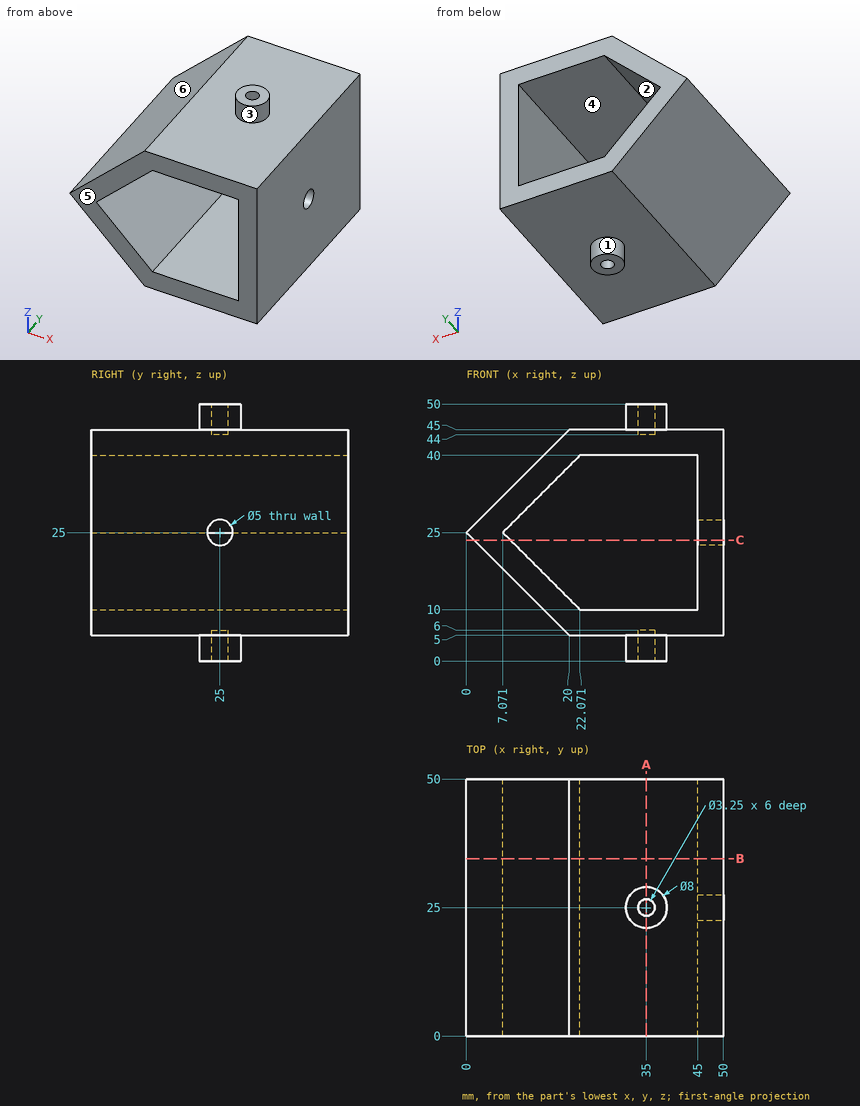
Verification items for this drawing (mm, ordinates from the low corner). A direction names the side the tool comes from. Give positions to 0.01 mm unless a question says otherwise; leave off trailing zeros. Loops run counter-clockwise (first coordinate to the right, second up) from the corner with the lowest first, then second, coordinate; pieces in that order, holes last.
1. Cross-section at A-A on x = 35. Record the cut outline in (y, z) (3 decimals), and give its area (3 significant figures).
Derived:
outline: (0, 5) - (21, 5) - (21, 0) - (23.375, 0) - (23.375, 6) - (26.625, 6) - (26.625, 0) - (29, 0) - (29, 5) - (50, 5) - (50, 10) - (0, 10) - close; (0, 40) - (50, 40) - (50, 45) - (29, 45) - (29, 50) - (26.625, 50) - (26.625, 44) - (23.375, 44) - (23.375, 50) - (21, 50) - (21, 45) - (0, 45) - close
area: 541 mm2
2. Cross-section at B-B on y = 34.5. Record the cut outline in (x, z).
Derived:
outline: (0, 25) - (20, 5) - (50, 5) - (50, 45) - (20, 45) - close; hole (7.07, 25) - (22.07, 10) - (45, 10) - (45, 40) - (22.07, 40) - close
3. Material ranges on probe 1 along Y at (x, z) = (46.85, 25); probe 2 along Z at (x, y) = (30, 13); probe 3 along X at (y, z) = (25, 2.45) (3 decimals), recorded low to high.
Derived:
probe 1: y = 0 to 22.5, 27.5 to 50
probe 2: z = 5 to 10, 40 to 45
probe 3: x = 31 to 33.375, 36.625 to 39
4. Tool access check on the marked faces 1, 2 and 3. Record the directions out of +Z, -Z, +X, -X, +Y, -Y that give a thin tool (end or side, any length) a straight path to the whole face; none if there is none.
Derived:
face 1: -Z
face 2: +Y, -Y
face 3: +Z
5. Cross-section at C-C on z = 23.5. Record the cut outline in (x, y).
Derived:
outline: (1.5, 0) - (8.57, 0) - (8.57, 50) - (1.5, 50) - close; (45, 0) - (50, 0) - (50, 23) - (45, 23) - close; (45, 27) - (50, 27) - (50, 50) - (45, 50) - close
6. Go/stop test with flat-tipped pins: P1, Ø5, axis at x = 35, y = 25, coming from the +Z side; P2, Ø8, axis at x = 20, y = 36.5, coming from the +Z side; P3, Ø5, axis at x = 40.5, z = 22, coming from the -Y side; P4, Ø1.5, axis at y = 24.5, z = 41.5, coming from the -X side. Record where each tip stops, or that it passes through.
Derived:
P1: stops at z = 50
P2: stops at z = 45
P3: passes through
P4: stops at x = 15.75
7. Release check for a two-part mould opening along Z. For the marked faces 4, 5 and 6 record: +Z half, -Z half, draft (parallel to the pull), parting line (faces both ways), or undercut.
Derived:
face 4: undercut
face 5: draft
face 6: +Z half
